Study the drawing (mm; zero at the part's minimum x, y, z) and answer. A direction names the side the tool comes from. Coordinates: 2 decimals unless noted, no trailing zeros. Order: outer loops, then holes, each group sorted by start corner. A loop starts at its lowest first (then second) coordinate and runs counter-clockwise, first axis right, second up.
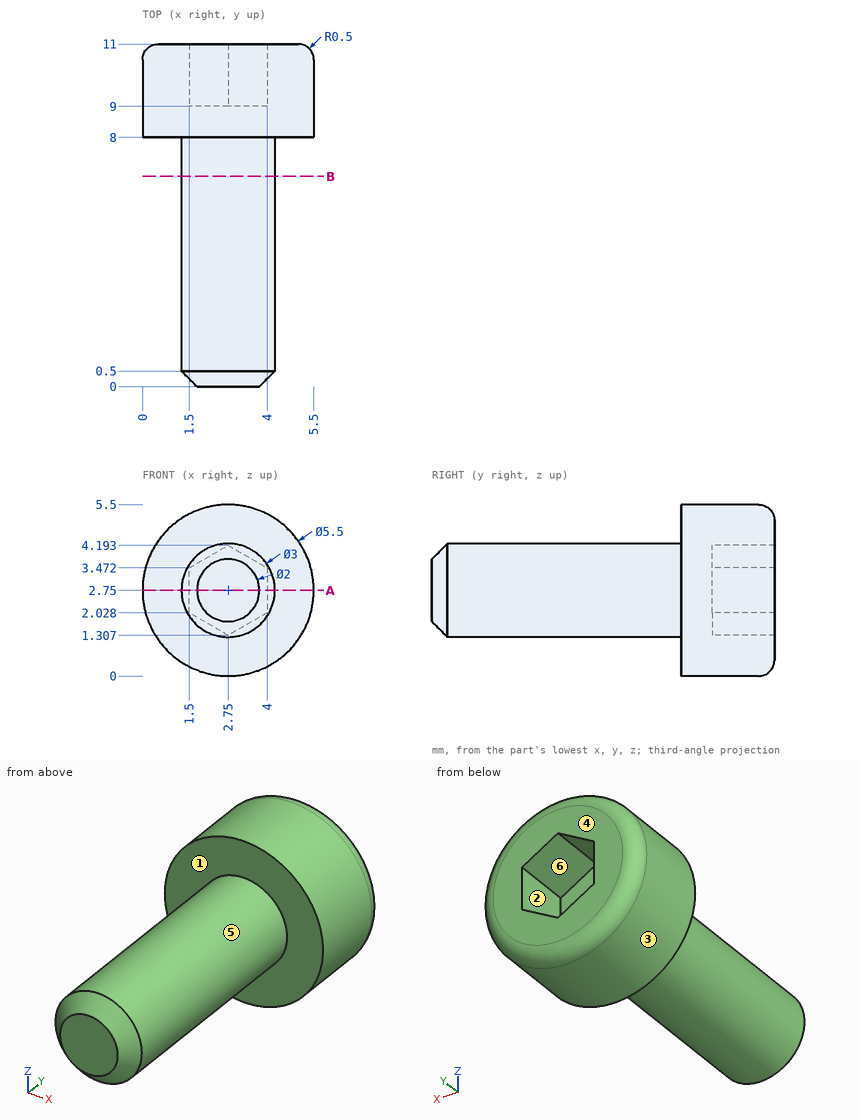
(1) The mould has two halves that part along Z. Classify the marked faces 4, 5 and 6: released by +Z, released by -Z, zero draft, split by the parting line, or undercut.
(2) Find section B-B (y = 6.75). Write down the section's boundary in (x, z).
(3) For the marked faces 1, 2 and 3, determine the directions among +Z, -Z, +X, -X, +Y, -Y from which every point of the face is accessible in a straight line to the end or side of a thin tool.
(4) This flat-tipped pin is pushed along its axis until it touches: pin 1 Ø1.5 at (y, z) = (3, 4) entering from +X (1 decimal). Where does it stop, or does it pass through?
(5) Consider line 1 (Y direction, x = 4.7, z = 3.4); line 2 (Y direction, x = 2.25, z = 2.3); line 3 (X direction, y = 5.75, z = 2.05). Determine where each line is inside the solid, lowest interval first.
(6) Find section A-A (z = 2.75). Write down the section's boundary in (x, y).
Findings below:
1. face 4: zero draft
1. face 5: split by the parting line
1. face 6: undercut
2. outline: circle Ø3 at (2.75, 2.75)
3. face 1: -Y
3. face 2: +Y
3. face 3: +Y, -Y
4. pin 1: stops at x = 4.2
5. line 1: y = 8 to 11
5. line 2: y = 0 to 9
5. line 3: x = 1.42 to 4.08
6. outline: (0, 8) - (1.25, 8) - (1.25, 0.5) - (1.75, 0) - (3.75, 0) - (4.25, 0.5) - (4.25, 8) - (5.5, 8) - (5.5, 10.5) arc R0.5 ccw to (5, 11) - (4, 11) - (4, 9) - (1.5, 9) - (1.5, 11) - (0.5, 11) arc R0.5 ccw to (0, 10.5) - close
